Read the model definition and answer for the solid it produces. Units are mm, in the model's axes. Round coordinates to 2 decimals unless told otherwise and drop trailing zeros. Write each loop counter-clockwise with the first axis right and the second up, starting at its lowest first coordinate (ties: lowest second). Pieces come first, ordered by that corner, then holes. Notation, with made-up numbers: (39, 35.5) - (55, 35.5) arc R21 ccw to (55, 60.5) - close; hole circle Ø1 at (20, -23). An arc over 180 degrees is marked (long way). Use one line per item in the form item = value. Start each with the question number.
1) Consider line 1 along Y through (x, z) = (-41, 24); line 2 along Z through (x, y) = (-50, 3); line 3 along Y through (x, z) = (-19.5, 34). Determine where each line is inside the solid, lowest interval first. Write a range as from..to.
2) For a pull along Y with two mould halves and no side action, classify faces 1 (the face through (-66, 25.344, 26)), 2 (the face through (-38.401, 22.034, 15.699)), 3 (the face through (-20.59, 25.75, 19.64)) as released by +Y, released by -Y, zero draft, split by the parting line, or undercut.
3) The part is cut by section A-A, the plane z = 17. Give the vertices of the cut face in (x, y), plus the area to 3 significant figures.
4) The part is cut by section C-C, the plane y = 11. Give the vertices of the cut face in (x, z), plus the area to 3 significant figures.
5) The part is cut by section B-B, the plane x = -57. Give the vertices of the cut face in (y, z), plus the area to 3 significant figures.
6) The part is cut by section D-D, the plane z = 20.25. Give the vertices of the cut face in (x, y), plus the area to 3 significant figures.
7) Each of these flat-tipped pins is pushed along its axis until it touches: pin 1 (5.5 mm diameter, centred on x = -37.4, z = 25.69, fed in from +Y); pin 2 (5.5 mm diameter, centred on x = -32.37, y = 13.63, fed in from +Z); pin 3 (12 mm diameter, centred on x = -36.5, y = 3.5, fed in from +Z). Where does it stop, or does it pass through?
from build123d import *

# Parameters (mm, degrees)
SKETCH1_W           = 20
SKETCH1_H           = 20
BOSS_EXTRUDE1_DEPTH = 0.8
SKETCH2_W           = 20
SKETCH2_H           = 0.8
BOSS_EXTRUDE2_DEPTH = 30
SKETCH3_W           = 5.674043307
SKETCH3_H           = 20
BOSS_EXTRUDE3_DEPTH = 0.8
SKETCH4_W           = 1.528315809
SKETCH4_H           = 5.562769748
CUT_EXTRUDE1_DEPTH  = 0.8
SKETCH5_W           = 4.145727498
SKETCH5_H           = 0.8
BOSS_EXTRUDE4_DEPTH = 20
SKETCH6_R           = 5
SKETCH6_R_2         = 1.65
CUT_EXTRUDE2_DEPTH  = 20
SKETCH7_R           = 5
SKETCH7_R_2         = 1.65
CUT_EXTRUDE3_DEPTH  = 20
SKETCH8_R           = 1.65
CUT_EXTRUDE4_DEPTH  = 50


with BuildPart() as part:
    # Sketch1 → Boss-Extrude1 (new body)
    with BuildSketch(Plane(origin=(0, 0, 0), x_dir=(1, 0, 0), z_dir=(0, 1, 0))):
        with Locations((-32.618726592, -25.293632959)):
            Rectangle(SKETCH1_W, SKETCH1_H)
    extrude(amount=BOSS_EXTRUDE1_DEPTH)

    # Sketch2 → Boss-Extrude2 (add)
    with BuildSketch(Plane(origin=(0, 0.8, 0), x_dir=(1, 0, 0), z_dir=(0, 1, 0))):
        with Locations((-32.618726592, -15.693632959)):
            Rectangle(SKETCH2_W, SKETCH2_H)
    extrude(amount=BOSS_EXTRUDE2_DEPTH)

    # Sketch3 → Boss-Extrude3 (add)
    with BuildSketch(Plane.XY.offset(16.093632959)):
        with Locations((-19.781704938, 16.144118187)):
            Rectangle(SKETCH3_W, SKETCH3_H)
    extrude(amount=-BOSS_EXTRUDE3_DEPTH)

    # Sketch4 → Cut-Extrude1 (cut)
    with BuildSketch(Plane.XY.offset(16.093632959)):
        with Locations((-21.854568688, 23.362733313)):
            Rectangle(SKETCH4_W, SKETCH4_H)
    extrude(amount=-CUT_EXTRUDE1_DEPTH, mode=Mode.SUBTRACT)

    # Sketch5 → Boss-Extrude4 (add)
    with BuildSketch(Plane.XY.offset(16.093632959)):
        with Locations((-19.017547034, 25.744118187)):
            Rectangle(SKETCH5_W, SKETCH5_H)
    extrude(amount=BOSS_EXTRUDE4_DEPTH)

    # Sketch6 → Cut-Extrude2 (cut)
    with BuildSketch(Plane.XY.offset(16.093632959)):
        with Locations((-32.374776475, 20.643164179)):
            Circle(SKETCH6_R)
        with Locations((-25.427511767, 20.643164179)):
            Circle(SKETCH6_R_2)
        with Locations((-32.2953483, 27.767794826)):
            Circle(SKETCH6_R_2)
        with Locations((-32.374776475, 13.629579794)):
            Circle(SKETCH6_R_2)
        with Locations((-39.287728189, 20.643164179)):
            Circle(SKETCH6_R_2)
        with Locations((-18.792512275, 20.600265825)):
            Circle(SKETCH6_R_2)
    extrude(amount=-CUT_EXTRUDE2_DEPTH, mode=Mode.SUBTRACT)

    # Mirror1: part across plane


with BuildPart() as part_1:
    add(part.part)
    add(part.part.mirror(Plane(origin=(-42.618726592, 0.8, 15.293632959), x_dir=(0, 0, 1), z_dir=(1, 0, 0))))

    # Sketch7 → Cut-Extrude3 (cut)
    with BuildSketch(Plane.XY.offset(16.093632959)):
        with Locations((-42.753979006, 9.78162079)):
            Circle(SKETCH7_R)
        with Locations((-42.833089812, 16.852996437)):
            Circle(SKETCH7_R_2)
        with Locations((-35.716428425, 9.860731596)):
            Circle(SKETCH7_R_2)
        with Locations((-49.875113272, 9.900286998)):
            Circle(SKETCH7_R_2)
        with Locations((-42.793534409, 2.818708136)):
            Circle(SKETCH7_R_2)
    extrude(amount=-CUT_EXTRUDE3_DEPTH, mode=Mode.SUBTRACT)

    # Sketch8 → Cut-Extrude4 (cut)
    with BuildSketch(Plane(origin=(0, 26.144118187, 0), x_dir=(1, 0, 0), z_dir=(0, 1, 0))):
        with Locations(Location((-66.255888471, -19.975736512, 0), (0, 0, 270))):
            Circle(SKETCH8_R)
        with Locations(Location((-66.255888471, -30.5502563, 0), (0, 0, 270))):
            Circle(SKETCH8_R)
        with Locations(Location((-18.981564713, -19.999660765, 0), (0, 0, 270))):
            Circle(SKETCH8_R)
        with Locations(Location((-18.981564713, -30.574180553, 0), (0, 0, 270))):
            Circle(SKETCH8_R)
        with Locations(Location((-53.863125461, -20.120296701, 0), (0, 0, 270))):
            Circle(SKETCH8_R)
        with Locations(Location((-53.863125461, -30.694816488, 0), (0, 0, 270))):
            Circle(SKETCH8_R)
        with Locations(Location((-32.905479909, -20.120296701, 0), (0, 0, 270))):
            Circle(SKETCH8_R)
        with Locations(Location((-32.905479909, -30.694816488, 0), (0, 0, 270))):
            Circle(SKETCH8_R)
        with Locations(Location((-57.872940418, -24.916981338, 0), (0, 0, 270))):
            Circle(SKETCH8_R)
        with Locations(Location((-49.389566156, -24.835777395, 0), (0, 0, 270))):
            Circle(SKETCH8_R)
        with Locations(Location((-37.40026466, -25.692156073, 0), (0, 0, 270))):
            Circle(SKETCH8_R)
        with Locations(Location((-29.147888307, -25.341819341, 0), (0, 0, 270))):
            Circle(SKETCH8_R)
    extrude(amount=-CUT_EXTRUDE4_DEPTH, mode=Mode.SUBTRACT)


solid = part_1.part
Geometry results:
q1.line_1 = 0..0.8
q1.line_2 = 15.29..16.09
q1.line_3 = 25.34..26.14
q2.face_1 = released by -Y
q2.face_2 = undercut
q2.face_3 = zero draft
q3.outline = (-68.29, 25.34) - (-64.15, 25.34) - (-64.15, 26.14) - (-68.29, 26.14) - close; (-62.62, 0) - (-22.62, 0) - (-22.62, 0.8) - (-62.62, 0.8) - close; (-21.09, 25.34) - (-16.94, 25.34) - (-16.94, 26.14) - (-21.09, 26.14) - close
q3.area = 38.6 mm2
q4.outline = (-68.29, 15.29) - (-51.11, 15.29) - (-51.11, 16.09) - (-68.29, 16.09) - close; (-48.65, 15.29) - (-47.6, 15.29) - (-47.6, 16.09) - (-48.65, 16.09) - close; (-37.9, 15.29) - (-36.91, 15.29) - (-36.91, 16.09) - (-37.9, 16.09) - close; (-34.52, 15.29) - (-16.94, 15.29) - (-16.94, 16.09) - (-34.52, 16.09) - close
q4.area = 29.4 mm2
q5.outline = (0, 15.29) - (17.84, 15.29) - (17.84, 16.09) - (0.8, 16.09) - (0.8, 23.52) - (0, 23.52) - close; (0, 26.32) - (0.8, 26.32) - (0.8, 35.29) - (0, 35.29) - close; (23.45, 15.29) - (30.8, 15.29) - (30.8, 16.09) - (23.45, 16.09) - close
q5.area = 33.3 mm2
q6.outline = (-68.29, 25.34) - (-67.88, 25.34) - (-67.88, 26.14) - (-68.29, 26.14) - close; (-64.63, 25.34) - (-64.15, 25.34) - (-64.15, 26.14) - (-64.63, 26.14) - close; (-62.62, 0) - (-55.51, 0) - (-55.51, 0.8) - (-62.62, 0.8) - close; (-52.22, 0) - (-34.55, 0) - (-34.55, 0.8) - (-52.22, 0.8) - close; (-31.26, 0) - (-22.62, 0) - (-22.62, 0.8) - (-31.26, 0.8) - close; (-21.09, 25.34) - (-20.61, 25.34) - (-20.61, 26.14) - (-21.09, 26.14) - close; (-17.35, 25.34) - (-16.94, 25.34) - (-16.94, 26.14) - (-17.35, 26.14) - close
q6.area = 28.2 mm2
q7.pin_1 = 0.8
q7.pin_2 = 16.09
q7.pin_3 = 35.29
